Source: CAD feature listing. Evaluate the final solid. Frame: model axes, mm. A direction names the side the tool comes from. Coordinates: 2 decimals unless noted, no trailing zeros. Order: outer loops, then holes, each group sorted by start corner. A loop starts at its lowest first (then second) coordinate and runs counter-clockwise, first axis right, second up.
Item 1: Ray query, line 1 (X direction, y = -0.25, z = 1); line 2 (X direction, y = -5.25, z = 1.25); line 3 (Y direction, x = -10.75, z = 1.5). Return the intervals inside material, ascending.
Item 2: Section C-C on y = -3.75. Return the cut outline in (x, z).
Item 3: Contact query for flat-ended pins moving along their axis: P1, Ø1, axis at x = -2, z = 3, coming from the -Y side; P2, Ø0.6, axis at x = -3.5, z = 2, coming from the -Y side; P3, Ø3.5, axis at y = -4, z = 2, coming from the +X side. Output: stop coordinate, or through.
Item 4: Section A-A on y = -6. Return the cut outline in (x, z), then the cut area to 3 significant figures.
Item 5: Section B-B on z = 2.5. Return the cut outline in (x, y), then the cut area to 3 significant figures.
Item 6: Reachability of faces 1 (the flat face through (-14, -4, 3)), 2 (the flat face through (-4.05, -1, 3)), 3 (the flat face through (-12, -3, 3)), 4 (the flat face through (11.988, 0, 3)), 5 (the flat face through (-11, -7.95, 3)) from +Z, -Z, +X, -X, +Y, -Y: full face, straight path, thin tool, end or side. Return the list, or none.
Item 7: Section D-D on x = 3.5. Return the cut outline in (y, z), then the cut area to 3 significant figures.
Item 8: Mould query, pull axis X, two halves, no side actions, for faces 6 (the flat face through (-12, -10, 3)), 7 (the flat face through (-3.5, -5, 3)), 8 (the flat face through (-5, -1, 0)), 9 (the flat face through (-3, 0, 3)). Classes: released by +X, released by -X, zero draft, split by the parting line, or undercut.
from build123d import *

# Parameters (mm, degrees)
F1_DEPTH = 7


with BuildPart() as f1:
    # F0 (on Top) → F1 (new body)
    with BuildSketch(Plane.XY):
        Polygon((-0.9, -7.4), (-0.9, 0), (-2.8, 0), (-2.8, -3.200004), (-2.8, -7.4), align=None)
        Polygon((-2.8, 0), (-0.9, 0), (10.1, 0), (10.1, -1.5), (11.988339, -1.5), (11.988339, 2), (0, 2), (-5.55, 2), (-5.55, 0), (-5.55, -2), (-4.05, -2), (-4.05, 0), align=None)
        Polygon((-2.8, -7.4), (-2.8, -3.200004), (-3.5, -4.300002), (-3.5, -6.300002), align=None)
        Polygon((-12, 0), (-5.55, 0), (-5.55, 2), (-14, 2), (-14, -6.45), (-12, -6.45), align=None)
        Polygon((-10, -6.45), (-12, -6.45), (-14, -6.45), (-14, -11.1), (-12, -11.1), (-12, -9.2), (-12, -7.95), (-10, -7.95), align=None)
    extrude(amount=F1_DEPTH)


solid = f1.part
Answer list:
1. line 1: x = -14 to -12, -5.55 to -4.05, -2.8 to -0.9, 10.1 to 11.99
1. line 2: x = -14 to -12, -3.5 to -0.9
1. line 3: y = -7.95 to -6.45, 0 to 2
2. outline: (-14, 0) - (-12, 0) - (-12, 7) - (-14, 7) - close; (-3.15, 0) - (-0.9, 0) - (-0.9, 7) - (-3.15, 7) - close
3. P1: stops at y = -7.4
3. P2: stops at y = -6.77
3. P3: stops at x = -0.9
4. outline: (-14, 0) - (-12, 0) - (-12, 7) - (-14, 7) - close; (-3.5, 0) - (-0.9, 0) - (-0.9, 7) - (-3.5, 7) - close
4. area: 32.2 mm2
5. outline: (-14, -11.1) - (-12, -11.1) - (-12, -7.95) - (-10, -7.95) - (-10, -6.45) - (-12, -6.45) - (-12, 0) - (-5.55, 0) - (-5.55, -2) - (-4.05, -2) - (-4.05, 0) - (-2.8, 0) - (-2.8, -3.2) - (-3.5, -4.3) - (-3.5, -6.3) - (-2.8, -7.4) - (-0.9, -7.4) - (-0.9, 0) - (10.1, 0) - (10.1, -1.5) - (11.99, -1.5) - (11.99, 2) - (-14, 2) - close
5. area: 99.2 mm2
6. face 1: +Z, -Z, -X, +Y, -Y
6. face 2: +Z, -Z, -Y
6. face 3: +Z, -Z
6. face 4: +Z, -Z, +X, +Y, -Y
6. face 5: +Z, -Z, +X, -Y
7. outline: (0, 0) - (2, 0) - (2, 7) - (0, 7) - close
7. area: 14.0 mm2
8. face 6: released by +X
8. face 7: undercut
8. face 8: zero draft
8. face 9: undercut
